```python
from build123d import *

# Parameters (mm, degrees)
SKETCH_1_W                       = 30
SKETCH_1_H                       = 35
EXTRUDE_1_DEPTH                  = 0.75
SKETCH_2_R                       = 1.05
CUT_EXTRUDE_1_DEPTH              = 1.5
EXTRUDE_2_DEPTH                  = 2.1
SKETCH_4_W                       = 3.5
SKETCH_4_H                       = 7.3
SKETCH_4_W_2                     = 7.3
SKETCH_4_H_2                     = 3.5
EXTRUDE_3_DEPTH                  = 5
SKETCH_5_W                       = 7.3
SKETCH_5_H                       = 3.5
EXTRUDE_4_DEPTH                  = 5
PATTERN_LINEAR_1_COUNT           = 2
PATTERN_LINEAR_1_PITCH           = 9
PATTERN_LINEAR_2_COUNT           = 3
PATTERN_LINEAR_2_PITCH           = 8
PATTERN_LINEAR_2_COPY_1_SKETCH_W = 7.3
PATTERN_LINEAR_2_COPY_1_SKETCH_H = 3.5
PATTERN_LINEAR_2_COPY_1_DEPTH    = 5
PATTERN_LINEAR_2_COPY_2_SKETCH_W = 7.3
PATTERN_LINEAR_2_COPY_2_SKETCH_H = 3.5
PATTERN_LINEAR_2_COPY_2_DEPTH    = 5
SKETCH_6_W                       = 3
SKETCH_6_H                       = 8
EXTRUDE_5_DEPTH                  = 4.5
SKETCH_7_W                       = 8
SKETCH_7_H                       = 20
EXTRUDE_6_DEPTH                  = 10


with BuildPart() as part:
    # ｽｹｯﾁ1 → ﾎﾞｽ - 押し出し1 (new, symmetric)
    with BuildSketch(Plane(origin=(0, 0, 0), x_dir=(1, 0, 0), z_dir=(0, 1, 0))):
        Rectangle(SKETCH_1_W, SKETCH_1_H)
    extrude(amount=EXTRUDE_1_DEPTH, both=True)

    # ｽｹｯﾁ2 → ｶｯﾄ - 押し出し1 (cut)
    with BuildSketch(Plane.XZ.offset(0.75)):
        with Locations(Location((-12.5, 15, 0), (0, 0, 270))):
            Circle(SKETCH_2_R)
        with Locations(Location((-12.5, -15, 0), (0, 0, 270))):
            Circle(SKETCH_2_R)
        with Locations(Location((12.5, 15, 0), (0, 0, 270))):
            Circle(SKETCH_2_R)
        with Locations(Location((12.5, -15, 0), (0, 0, 270))):
            Circle(SKETCH_2_R)
    extrude(amount=-CUT_EXTRUDE_1_DEPTH, mode=Mode.SUBTRACT)

    # ｽｹｯﾁ3 → ﾎﾞｽ - 押し出し2 (add)
    with BuildSketch(Plane.XZ.offset(0.75)):
        Polygon((-10, 17.5), (-10, 13.5), (-15, 13.5), (-15, -12.5), (-10, -12.5), (-10, -17.5), (10, -17.5), (10, -12.5), (15, -12.5), (15, 12.5), (10, 12.5), (10, 17.5), align=None)
    extrude(amount=EXTRUDE_2_DEPTH)

    # ｽｹｯﾁ4 → ﾎﾞｽ - 押し出し3 (add)
    with BuildSketch(Plane(origin=(0, 0.75, 0), x_dir=(1, 0, 0), z_dir=(0, 1, 0))):
        with Locations((5.25, 12.85)):
            Rectangle(SKETCH_4_W, SKETCH_4_H)
        with Locations((5.85, -14.75)):
            Rectangle(SKETCH_4_W_2, SKETCH_4_H_2)
    extrude(amount=EXTRUDE_3_DEPTH)

    # ｽｹｯﾁ5 → ﾎﾞｽ - 押し出し4 (add)
    with BuildSketch(Plane(origin=(0, 0.75, 0), x_dir=(1, 0, 0), z_dir=(0, 1, 0))):
        with Locations((-10.35, 11.25)):
            Rectangle(SKETCH_5_W, SKETCH_5_H)
    extrude_4 = extrude(amount=EXTRUDE_4_DEPTH)

    # 直線ﾊﾟﾀｰﾝ1: ﾎﾞｽ - 押し出し4 ×2
    with Locations(*[(i * PATTERN_LINEAR_1_PITCH, 0, 0) for i in range(1, PATTERN_LINEAR_1_COUNT)]):
        add(extrude_4)

    # 直線ﾊﾟﾀｰﾝ2: ﾎﾞｽ - 押し出し4 ×3
    with Locations(*[(0, 0, i * PATTERN_LINEAR_2_PITCH) for i in range(1, PATTERN_LINEAR_2_COUNT)]):
        add(extrude_4)

    # 直線ﾊﾟﾀｰﾝ2 copy 1 sketch → 直線ﾊﾟﾀｰﾝ2 copy 1 (add)
    with BuildSketch(Plane(origin=(9, 0.75, 8), x_dir=(1, 0, 0), z_dir=(0, 1, 0))):
        with Locations((-10.35, 11.25)):
            Rectangle(PATTERN_LINEAR_2_COPY_1_SKETCH_W, PATTERN_LINEAR_2_COPY_1_SKETCH_H)
    extrude(amount=PATTERN_LINEAR_2_COPY_1_DEPTH)

    # 直線ﾊﾟﾀｰﾝ2 copy 2 sketch → 直線ﾊﾟﾀｰﾝ2 copy 2 (add)
    with BuildSketch(Plane(origin=(9, 0.75, 16), x_dir=(1, 0, 0), z_dir=(0, 1, 0))):
        with Locations((-10.35, 11.25)):
            Rectangle(PATTERN_LINEAR_2_COPY_2_SKETCH_W, PATTERN_LINEAR_2_COPY_2_SKETCH_H)
    extrude(amount=PATTERN_LINEAR_2_COPY_2_DEPTH)

    # ｽｹｯﾁ6 → ﾎﾞｽ - 押し出し5 (add)
    with BuildSketch(Plane(origin=(0, 0.75, 0), x_dir=(1, 0, 0), z_dir=(0, 1, 0))):
        with Locations((12.5, 6.5)):
            Rectangle(SKETCH_6_W, SKETCH_6_H)
    extrude(amount=EXTRUDE_5_DEPTH)

    # ｽｹｯﾁ7 → ﾎﾞｽ - 押し出し6 (add)
    with BuildSketch(Plane(origin=(0, 0.75, 0), x_dir=(1, 0, 0), z_dir=(0, 1, 0))):
        with Locations((-6, -21.5)):
            Rectangle(SKETCH_7_W, SKETCH_7_H)
    extrude(amount=EXTRUDE_6_DEPTH)


solid = part.part
```
Work out the finished part from the listing and answer in its coordinate system (mm). A direction names the side the tool comes from. Give positions to 0.01 mm unless a question says otherwise; leave off trailing zeros. Write each loop counter-clockwise with the first axis right and the second up, starting at its lowest first coordinate (ties: lowest second). Pieces come first, ordered by that corner, then holes.
(1) The part is cut by section A-A on x = 12.5. Write down the section's boundary in (y, z), plus the area to 3 significant figures.
Final values:
outline: (-2.85, -12.5) - (-0.75, -12.5) - (-0.75, -13.95) - (0.75, -13.95) - (0.75, -10.5) - (5.25, -10.5) - (5.25, -2.5) - (0.75, -2.5) - (0.75, 13.95) - (-0.75, 13.95) - (-0.75, 12.5) - (-2.85, 12.5) - close; (-0.75, -17.5) - (0.75, -17.5) - (0.75, -16.05) - (-0.75, -16.05) - close; (-0.75, 16.05) - (0.75, 16.05) - (0.75, 17.5) - (-0.75, 17.5) - close
area: 135 mm2
(2) Which of the six approach directions +Z, -Z, +X, -X, +Y, -Y give full straight-line access (tool end or side, diameter ignored) to faces 5 (the flat face through (-6.7, 3, -3)), 6 (the flat face through (5, 3, -16.5)), 7 (the flat face through (-10, 6, 22)), 8 (the flat face through (5, 3, -9.2))?
Final values:
face 5: -Z, +Y
face 6: -Z, +X, -X, +Y
face 7: +Z, -X, +Y
face 8: -X, +Y
(3) Straight lines are drawn through the part: line 1 (X direction, y = 4, z = -3); line 2 (X direction, y = 0.45, z = 15); line 3 (Z direction, x = -4, y = 1.75). For each, find the intervals that lie inside material, in ascending order.
Final values:
line 1: x = -14 to -6.7, -5 to 2.3, 11 to 14
line 2: x = -15 to -13.55, -11.45 to 11.45, 13.55 to 15
line 3: z = -13 to -9.5, -5 to -1.5, 3 to 6.5, 11.5 to 31.5
(4) The part is cut by section C-C on y = -1.5. Write down the section's boundary in (x, z), plus the area to 3 significant figures.
Final values:
outline: (-15, -12.5) - (-10, -12.5) - (-10, -17.5) - (10, -17.5) - (10, -12.5) - (15, -12.5) - (15, 12.5) - (10, 12.5) - (10, 17.5) - (-10, 17.5) - (-10, 13.5) - (-15, 13.5) - close
area: 955 mm2
(5) Flat-ended cylindrical pins translate along their axes: pin 1 Ø1 at (x, z) = (-10.5, -11.5) entering from +Y; pin 2 Ø3.5 at (x, z) = (12, -5) entering from +Y; pin 3 Ø2.5 at (x, y) = (-9, 2.5) entering from -Z. Find the tip coordinate at first contact, or state that the pin passes through.
Final values:
pin 1: stops at y = 5.75
pin 2: stops at y = 5.25
pin 3: stops at z = -13
(6) The part is cut by section B-B on z = -15. Write down the section's boundary in (x, y).
Final values:
outline: (-15, -0.75) - (-13.55, -0.75) - (-13.55, 0.75) - (-15, 0.75) - close; (-11.45, -0.75) - (-10, -0.75) - (-10, -2.85) - (10, -2.85) - (10, -0.75) - (11.45, -0.75) - (11.45, 0.75) - (7, 0.75) - (7, 5.75) - (3.5, 5.75) - (3.5, 0.75) - (-11.45, 0.75) - close; (13.55, -0.75) - (15, -0.75) - (15, 0.75) - (13.55, 0.75) - close
(7) The part is cut by section D-D on x = 0. Write down the section's boundary in (y, z), plus the area to 4 significant figures.
Final values:
outline: (-2.85, -17.5) - (0.75, -17.5) - (0.75, -13) - (5.75, -13) - (5.75, -9.5) - (0.75, -9.5) - (0.75, -5) - (5.75, -5) - (5.75, -1.5) - (0.75, -1.5) - (0.75, 3) - (5.75, 3) - (5.75, 6.5) - (0.75, 6.5) - (0.75, 17.5) - (-2.85, 17.5) - close
area: 178.5 mm2
(8) The mould has two halves that part along X. Classify faces 1 (the flat face through (-5, 3, -3)), 2 (the flat face through (6, 5.75, 15)), 3 (the flat face through (15, -1, 0)), 4 (the flat face through (-14, 3, 5)): pulls with the +X half, pulls with the -X half, needs draft (parallel to the pull), parting line crosses it, or undercut.
Final values:
face 1: undercut
face 2: needs draft
face 3: pulls with the +X half
face 4: pulls with the -X half
